Design review of the part shown in the three views and the two pictorial views. Dimensions are in mm from the part's minimum x, y and z. A direction names the side the tool comes from. Coordinates: 2 decimals unless noted, no trailing zeros. Loops run counter-clockwise (first coordinate to the right, second up) from the corner with the lowest first, then second, coordinate; pieces in that order, holes last. Notation, with made-up numbers: (-24, 21.25) -> (18, 21.25) arc R13 ccw to (18, 30.25) -> close; hole circle Ø5 at (62.5, 3). An arc over 180 degrees is marked (long way). Use a Markdown table: item, result. Add a question column.
Q1. Take a section at C-C on y = 18. Write out the cut boundary in (x, z).
Q2. Draft analysis for pull direction X (two halves, no side actions). For the marked faces 4, 5 and 6, state which applies: pulls with the +X half, pulls with the -X half, needs draft (parallel to the pull), parting line crosses it, or undercut.
Q3. For probe 1 along Y at (x, z) = (38, 4); probe 2 along Y at (x, z) = (19, 7), list the stretches that pass through material, from the lowest coordinate up.
Q4. For the marked faces 1, 2 and 3, list the 3-axis set-ups (+Z, -Z, +X, -X, +Y, -Y) from which the entire face can be reached by the end or side of a thin tool; tool diameter is ignored.
Q5. Take a section at D-D on x = 19.05. Write out the cut boundary in (y, z) (3 decimals), plus the area to 3 significant figures.
Q6. Clearance check with flat-ended pins moving along their axes: pin 1 Ø4 at (y, z) = (51.5, 7.5) entering from +X; pin 2 Ø10 at (x, z) = (23, 4.5) entering from -Y; pin 3 Ø4 at (x, z) = (23.5, 4) entering from +Y. State where each tip first meets the part, or that it passes through.
Q7. Take a section at A-A on y = 38.1. Write out the cut boundary in (x, z) (1 decimal), plus the area to 3 significant figures.
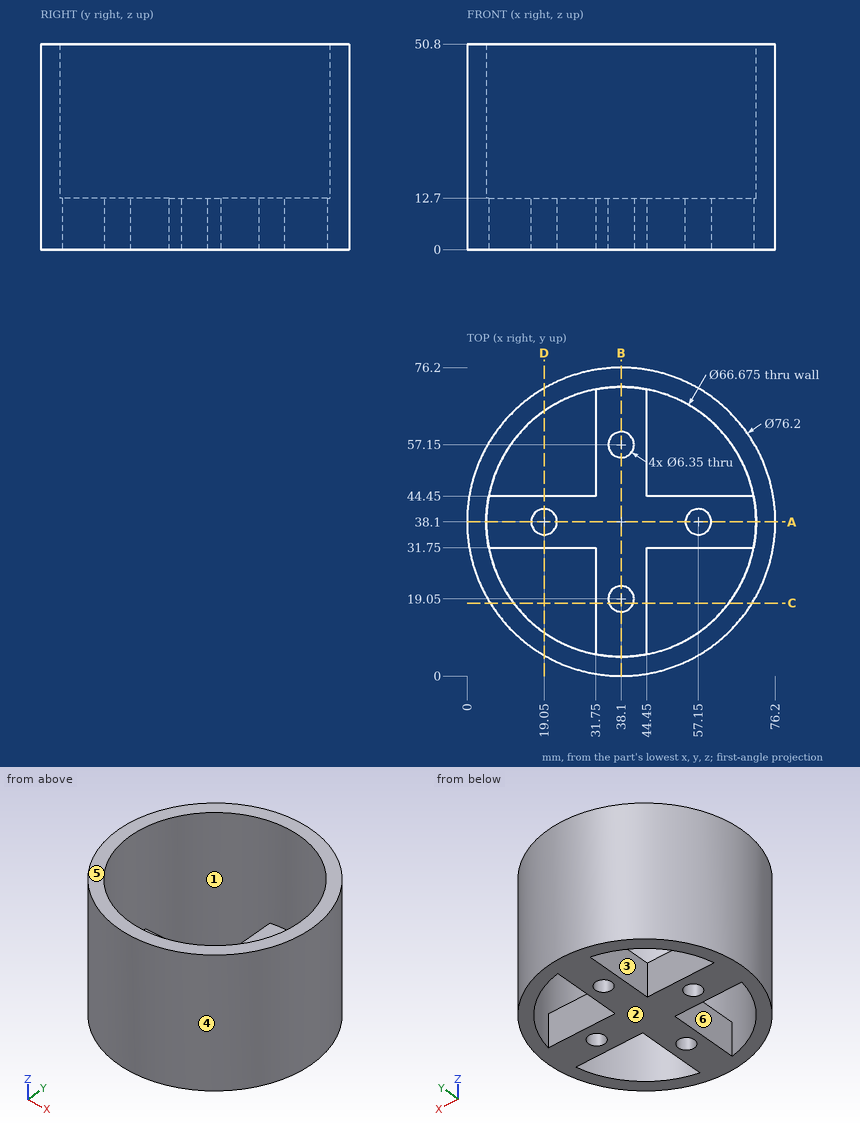
Answer list:
| question | item | result |
|---|---|---|
| 1 | outline | (5.73, 0) -> (11.5, 0) -> (11.5, 50.8) -> (5.73, 50.8) -> close; (31.75, 0) -> (35.1, 0) -> (35.1, 12.7) -> (31.75, 12.7) -> close; (41.1, 0) -> (44.45, 0) -> (44.45, 12.7) -> (41.1, 12.7) -> close; (64.7, 0) -> (70.47, 0) -> (70.47, 50.8) -> (64.7, 50.8) -> close |
| 2 | face 4 | parting line crosses it |
| 2 | face 5 | needs draft |
| 2 | face 6 | undercut |
| 3 | probe 1 | 0 to 15.88, 22.22 to 53.98, 60.32 to 76.2 |
| 3 | probe 2 | 5.13 to 10.78, 31.75 to 34.93, 41.27 to 44.45, 65.42 to 71.07 |
| 4 | face 1 | +Z |
| 4 | face 2 | -Z, +X, -X, +Y, -Y |
| 4 | face 3 | +Z, -Z |
| 5 | outline | (5.104, 0) -> (10.742, 0) -> (10.742, 50.8) -> (5.104, 50.8) -> close; (31.75, 0) -> (34.925, 0) -> (34.925, 12.7) -> (31.75, 12.7) -> close; (41.275, 0) -> (44.45, 0) -> (44.45, 12.7) -> (41.275, 12.7) -> close; (65.458, 0) -> (71.096, 0) -> (71.096, 50.8) -> (65.458, 50.8) -> close |
| 5 | area | 653 mm² |
| 6 | pin 1 | x = 74.45 |
| 6 | pin 2 | y = 1.36 |
| 6 | pin 3 | y = 74.06 |
| 7 | outline | (0, 0) -> (15.9, 0) -> (15.9, 12.7) -> (4.8, 12.7) -> (4.8, 50.8) -> (0, 50.8) -> close; (22.2, 0) -> (54, 0) -> (54, 12.7) -> (22.2, 12.7) -> close; (60.3, 0) -> (76.2, 0) -> (76.2, 50.8) -> (71.4, 50.8) -> (71.4, 12.7) -> (60.3, 12.7) -> close |
| 7 | area | 1,170 mm² |
